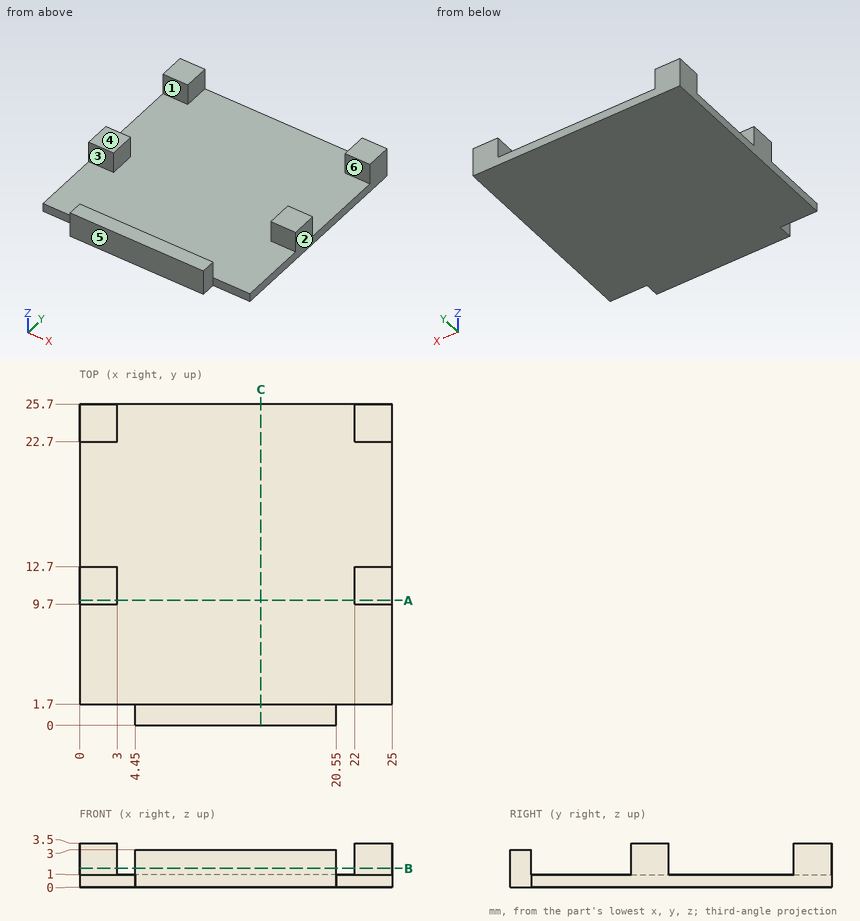
Geometry check sheet. Reference: drawing and pictorial views, mm from the part's lowest x, y, z. A direction names the side the tool comes from. Give positions to 0.01 mm unless a question says otherwise; leave off trailing zeros. Order: outer loops, then holes, each group sorted by start corner. A loop starts at its lowest first (then second) coordinate and runs counter-clockwise, first axis right, second up. Notation, with made-up numbers: M -6.5,17 L 4.5,17 A14 ccw 4.5,27 Z; hole C -6.75,-14.75 d11. An arc over 180 degrees is marked long. Answer as a JSON object with one key per item and string values. Group by question number.
1) Depth check by flat-ended pin: pin 1 Ø0.8 at (x, z) = (22, 0.5) entering from -Y; pin 2 Ø1.9 at (y, z) = (1, 1.5) entering from -X; pin 3 Ø0.5 at (y, z) = (0.5, 2) entering from +X; pin 4 Ø2 at (x, z) = (24, 2.5) entering from -Y. Enter the tip coordinate at first touch or a pass-through.
2) Mould release check, pull along Y, two halves, no side actions. Record for the marked faces 4, 5 and 6: released by +Y, released by -Y, zero draft, split by the parting line, or undercut.
3) Access from +Z, -Z, +X, -X, +Y, -Y to the whole of each face (thin tool, end or side, straight path). Record for the marked faces 1, 2 and 3.
4) Cross-section at B-B (z = 1.5). Enter the section's corners in (x, y).
5) Cross-section at C-C (x = 14.5). Enter the section's corners in (y, z), then the cut area to 3 significant figures.
6) Scan lines: line 1 along Y through (x, z) = (2.75, 3.1); line 2 along X through (y, z) = (9.75, 1.4); line 3 along Y through (x, z) = (20.75, 0.7). Record each from-to range of solid material in increasing order. Write a range as [from, to].
7) Cross-section at A-A (y = 10). Enter the section's corners in (x, z).
Result sheet:
{
 "1": {"pin 1": "stops at y = 1.7", "pin 2": "stops at x = 0", "pin 3": "stops at x = 20.55", "pin 4": "stops at y = 9.7"},
 "2": {"face 4": "zero draft", "face 5": "released by -Y", "face 6": "undercut"},
 "3": {"face 1": "+Z, +X, -X", "face 2": "+Z, -Z, +X, +Y, -Y", "face 3": "+Z, +X, -X, -Y"},
 "4": {"outline": "M 0,9.7 L 3,9.7 L 3,12.7 L 0,12.7 Z; M 0,22.7 L 3,22.7 L 3,25.7 L 0,25.7 Z; M 4.45,0 L 20.55,0 L 20.55,1.7 L 4.45,1.7 Z; M 22,9.7 L 25,9.7 L 25,12.7 L 22,12.7 Z; M 22,22.7 L 25,22.7 L 25,25.7 L 22,25.7 Z"},
 "5": {"outline": "M 0,0 L 25.7,0 L 25.7,1 L 1.7,1 L 1.7,3 L 0,3 Z", "area": "29.1 mm2"},
 "6": {"line 1": "y = [9.7, 12.7], [22.7, 25.7]", "line 2": "x = [0, 3], [22, 25]", "line 3": "y = [1.7, 25.7]"},
 "7": {"outline": "M 0,0 L 25,0 L 25,3.5 L 22,3.5 L 22,1 L 3,1 L 3,3.5 L 0,3.5 Z"}
}
